```python
from build123d import *

# Parameters (mm, degrees)
BOSS_EXTRUDE1_DEPTH  = 38.1
FILLET1_R            = 6.35
M5_CLEARANCE_HOLE1_D = 5.3


with BuildPart() as part:
    # Sketch1 → Boss-Extrude1 (new body)
    with BuildSketch(Plane.XY):
        Polygon((0, 0), (31.75, 0), (31.75, 6.35), (6.35, 6.35), (6.35, 31.75), (0, 31.75), align=None)
    extrude(amount=BOSS_EXTRUDE1_DEPTH)

    # Fillet1
    fillet1_edges = [part.edges().sort_by_distance(p)[0] for p in [
        (31.75, 6.35, 19.05),
        (6.35, 31.75, 19.05),
    ]]
    fillet(fillet1_edges, radius=FILLET1_R - 0.0001)  # a hair under: the kernel refuses the full size

    # M5 Clearance Hole1 (through all)
    with Locations(Plane(origin=(6.35, 0, 0), x_dir=(0, 0, -1), z_dir=(1, 0, 0))):
        with Locations((-31.75, 19.05), (-6.35, 19.05)):
            m5_clearance_hole1 = Hole(M5_CLEARANCE_HOLE1_D / 2)

    # Mirror1: M5 Clearance Hole1 across plane
    add(m5_clearance_hole1.mirror(Plane(origin=(0, 0, 0), x_dir=(0, 0, 1), z_dir=(-0.7071067811865472, 0.7071067811865479, 0))), mode=Mode.SUBTRACT)


solid = part.part
```
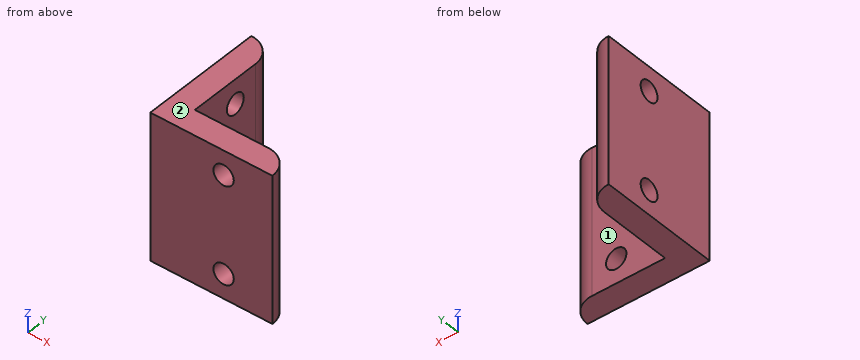
For this review, take the finished solid that the model builds, in its own axes (mm). Face numbers are marked on the shaded views. A direction names the side the tool comes from. Round coordinates to 2 decimals unless told otherwise and drop trailing zeros. Write each loop counter-clockwise with the first axis right and the second up, starting at its lowest first coordinate (ties: lowest second). Pieces come first, ordered by that corner, then holes.
1) Insertion check: pin 1 Ø12 at (x, z) = (9, 4.5) entering from +Y; pin 2 Ø1.5 at (x, y) = (4.5, 9.5) entering from -Z; pin 3 Ø8.5 at (x, z) = (19.05, 31.75) entering from +Y; pin 4 Ø8.5 at (y, z) = (19.05, 6.35) entering from +X. Each pin has a flat end and moves straight along its axis. Give the tip position at first contact, or say it passes through.
Answer below:
pin 1: stops at y = 31
pin 2: stops at z = 0
pin 3: stops at y = 6.35
pin 4: stops at x = 6.35
2) For line 1 along Y through (x, z) = (25.5, 24), list the stretches that pass through material, from the lowest coordinate up.
Answer below:
line 1: y = 0 to 6.35
3) Take a section at B-B on z = 6.35. State how many separate pieces and enclosed holes the cut face has, then the cut area to 3 significant figures.
Answer below:
separate pieces: 3
enclosed holes: 0
area: 278 mm2
4) Take a section at A-A on x = 19.05. Give the boundary of the cut face in (y, z).
Answer below:
outline: (0, 0) - (6.35, 0) - (6.35, 3.7) - (0, 3.7) - close; (0, 9) - (6.35, 9) - (6.35, 29.1) - (0, 29.1) - close; (0, 34.4) - (6.35, 34.4) - (6.35, 38.1) - (0, 38.1) - close
5) Machinability: for the marked faces 1 and 2, which of the approach directions +Z, -Z, +X, -X, +Y, -Y give a long, thin tool a straight path to every point of the face, cutting with its end or side? Answer none if there is none.
Answer below:
face 1: +Z, -Z, +X, +Y
face 2: +Z, +X, -X, +Y, -Y
